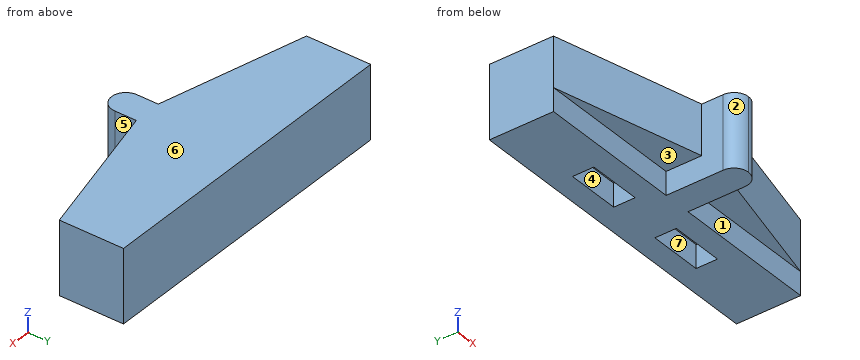
from build123d import *

# Parameters (mm, degrees)
SKETCH1_W           = 15
SKETCH1_H           = 6
SKETCH1_W_2         = 8
SKETCH1_H_2         = 20
BOSS_EXTRUDE1_DEPTH = 14
SKETCH3_W           = 15
SKETCH3_H           = 6
SKETCH3_W_2         = 8
SKETCH3_H_2         = 20
BOSS_EXTRUDE2_DEPTH = 6.5
FILLET1_R           = 4


with BuildPart() as part:
    # Sketch1 → Boss-Extrude1 (new body)
    # profile 1 of 6: a face of its own
    with BuildSketch(Plane.XY):
        Polygon((-4, -9), (4, -9), (45, -9), (45, 9), (-45, 9), (-45, -9), align=None)
        with Locations((-15, 0)):
            Rectangle(SKETCH1_W, SKETCH1_H, mode=Mode.SUBTRACT)
        with Locations((15, 0)):
            Rectangle(SKETCH1_W, SKETCH1_H, mode=Mode.SUBTRACT)
    # profile 2 of 6: a face of its own
    with BuildSketch(Plane.XY):
        with Locations((0, -19)):
            Rectangle(SKETCH1_W_2, SKETCH1_H_2)
    # profile 3 of 6: a face of its own
    with BuildSketch(Plane.XY):
        with Locations((-15, 0)):
            Rectangle(SKETCH1_W, SKETCH1_H)
    # profile 4 of 6: a face of its own
    with BuildSketch(Plane.XY):
        with Locations((15, 0)):
            Rectangle(SKETCH1_W, SKETCH1_H)
    # profile 5 of 6: a face of its own
    with BuildSketch(Plane.XY):
        Polygon((45, -9), (4, -9), (4, -19), align=None)
    # profile 6 of 6: a face of its own
    with BuildSketch(Plane.XY):
        Polygon((-4, -19), (-4, -9), (-45, -9), align=None)
    extrude(amount=BOSS_EXTRUDE1_DEPTH)

    # Sketch3 → Boss-Extrude2 (add)
    # profile 1 of 2: a face of its own
    with BuildSketch(Plane.XY):
        Polygon((-4, -9), (4, -9), (45, -9), (45, 9), (-45, 9), (-45, -9), align=None)
        with Locations((-15, 0)):
            Rectangle(SKETCH3_W, SKETCH3_H, mode=Mode.SUBTRACT)
        with Locations((15, 0)):
            Rectangle(SKETCH3_W, SKETCH3_H, mode=Mode.SUBTRACT)
    # profile 2 of 2: a face of its own
    with BuildSketch(Plane.XY):
        with Locations((0, -19)):
            Rectangle(SKETCH3_W_2, SKETCH3_H_2)
    extrude(amount=-BOSS_EXTRUDE2_DEPTH)

    # Fillet1
    fillet1_edges = [part.edges().sort_by_distance(p)[0] for p in [
        (-4, -29, 3.75),
        (4, -29, 3.75),
    ]]
    fillet(fillet1_edges, radius=FILLET1_R - 0.0001)  # a hair under: the kernel refuses the full size


solid = part.part
The model under review builds one solid part; all positions refer to its coordinate system, in mm. Face numbers are marked on the shaded views. A direction names the side the tool comes from. Round coordinates to 2 decimals unless told otherwise and drop trailing zeros. Write each loop counter-clockwise with the first axis right and the second up, starting at its lowest first coordinate (ties: lowest second). Pieces come first, ordered by that corner, then holes. Notation, with made-up numbers: M 86,5.5 L 92,5.5 A10 cw 92,14.5 Z; hole C 25,18.5 d7. An arc over 180 degrees is marked long. Use a Markdown table: item, result. Add a question column.
Q1. We need section B-B, the plane y = 2. State the section outline as (x, z) points, plus the area to 3 significant figures.
Q2. To check wall thickness, follow line 1 (Y direction, x = 17, z = -1.25); line 2 (X direction, y = -23.5, z = 12); line 3 (Y direction, x = -29, z = -1). State the ranges of each line that lie inside material, in increasing order.
Q3. Insertion check: pin 1 (2 mm diameter, centred on y = -23, z = 9.5, fed in from -X); pin 2 (3 mm diameter, centred on x = -17.5, y = -0.5, fed in from -Z); pin 3 (3 mm diameter, centred on x = 22.5, z = -3, fed in from -Y). Each pin has a flat end and moves straight along its axis. Give the tip position at first contact, or say it passes through.
Q4. The part is to be moulded in two halves that separate along X. For the marked faces 5, 6 and 7, say which applies: pulls with the +X half, pulls with the -X half, needs draft (parallel to the pull), parting line crosses it, or undercut.
Q5. Machinability: for the marked faces 1, 2, 3 and 4, which of the approach directions +Z, -Z, +X, -X, +Y, -Y give a long, thin tool a straight path to every point of the face, cutting with its end or side? Answer none if there is none.
Q6. We need section D-D, the plane x = -8.5. State the section outline as (y, z) points.
Q7. We need section A-A, the plane z = -5. Count the separate pieces of the cut face and the enclosed holes in it, plus the area to 3 significant figures.
Findings below:
| question | item | result |
|---|---|---|
| 1 | outline | M -45,-6.5 L -22.5,-6.5 L -22.5,0 L -7.5,0 L -7.5,-6.5 L 7.5,-6.5 L 7.5,0 L 22.5,0 L 22.5,-6.5 L 45,-6.5 L 45,14 L -45,14 Z |
| 1 | area | 1,650 mm² |
| 2 | line 1 | y = -9 to -3, 3 to 9 |
| 2 | line 2 | x = -4 to 4 |
| 2 | line 3 | y = -9 to 9 |
| 3 | pin 1 | stops at x = -4 |
| 3 | pin 2 | stops at z = 0 |
| 3 | pin 3 | stops at y = -9 |
| 4 | face 5 | pulls with the +X half |
| 4 | face 6 | needs draft |
| 4 | face 7 | undercut |
| 5 | face 1 | -Z, +X, -Y |
| 5 | face 2 | +Z, -Z, -X, -Y |
| 5 | face 3 | -Z, -X, -Y |
| 5 | face 4 | -Z |
| 6 | outline | M -17.9,0 L -9,0 L -9,-6.5 L -3,-6.5 L -3,0 L 3,0 L 3,-6.5 L 9,-6.5 L 9,14 L -17.9,14 Z |
| 7 | separate pieces | 1 |
| 7 | enclosed holes | 2 |
| 7 | area | 1,590 mm² |
